Autodesk Inventor part; units mm, degrees
ref_plane "YZ Plane" through (0, 0, 0) normal (1, 0, 0) x (0, 1, 0)
ref_plane "XZ Plane" through (0, 0, 0) normal (0, 1, 0) x (-1, 0, 0)
ref_plane "XY Plane" through (0, 0, 0) normal (0, 0, 1) x (1, 0, 0)
sketch "Sketch1" plane through (0, 0, 0) normal (0, 0, 1) x (1, 0, 0)
  line L0 (30, -30) -> (30, 30)
  line L1 (30, 30) -> (-30, 30)
  line L2 (-30, 30) -> (-30, -30)
  line L3 (-30, -30) -> (30, 30) construction
  line L4 (30, -30) -> (-30, 30) construction
  line L5 (30, 30) -> (25, 30) construction
  line L6 (25, 30) -> (25, 25) construction
  line L7 (-30, 30) -> (-25, 30) construction
  line L8 (-25, 30) -> (-25, 25) construction
  line L9 (-30, -30) -> (-30, -25) construction
  line L10 (-30, -25) -> (-25, -25) construction
  line L11 (30, -30) -> (30, -25) construction
  line L12 (30, -25) -> (25, -25) construction
  circle A0 centre (-25, 25) radius 1.5
  circle A1 centre (25, 25) radius 1.5
  circle A2 centre (25, -25) radius 1.5
  circle A3 centre (-25, -25) radius 1.5
  line L13 (30, 30) -> (30, 18) construction
  line L14 (30, 18) -> (-30, 18)
  point P0 (0, 0)
  dimension "d0" = 60
  dimension "d1" = 60
  dimension "d2" = 5
  dimension "d3" = 5
  dimension "d4" = 5
  dimension "d5" = 5
  dimension "d6" = 5
  dimension "d7" = 5
  dimension "d8" = 5
  dimension "d9" = 5
  dimension "d10" = 3
  dimension "d11" = 3
  dimension "d12" = 3
  dimension "d13" = 3
  dimension "d46" = 12
sketch "Sketch1 outline for Block" plane through (0, 0, 0) normal (0, 0, 1) x (1, 0, 0)
  line L0 (30, 30) -> (30, 18)
  line L1 (-30, 30) -> (30, 30)
  line L2 (30, 18) -> (-30, 18)
  line L3 (-30, 18) -> (-30, 30)
  circle A0 centre (-25, 25) radius 1.5
  circle A1 centre (25, 25) radius 1.5
extrude "Block" add sketch "Sketch1 outline for Block" along normal blind 60
sketch "Sketch2" plane through (30, -30, 0) normal (1, 0, 0) x (0, 0, -1)
  line L0 (0, 60) -> (-60, 60)
  line L1 (-30, 60) -> (-12.75, 60)
  line L2 (-30, 60) -> (-47.25, 60)
  line L3 (-30, 60) -> (-30, 51.1) construction
  line L4 (-30, 51.1) -> (-6.75, 51.1)
  line L5 (-30, 51.1) -> (-53.25, 51.1)
  line L6 (-53.25, 51.1) -> (-53.25, 53.1)
  line L7 (-6.75, 51.1) -> (-6.75, 53.1)
  line L8 (-6.75, 53.1) -> (-12.75, 60)
  line L9 (-53.25, 53.1) -> (-47.25, 60)
  point P0 (0, 30)
  dimension "d17" = 17.25
  dimension "d18" = 17.25
  dimension "d19" = 8.9
  dimension "d20" = 23.25
  dimension "d21" = 23.25
  dimension "d22" = 2
  dimension "d23" = 2
sketch "Sketch2 outline for Tripod Slot" plane through (30, -30, 0) normal (1, 0, 0) x (0, 0, -1)
  line L0 (-12.75, 60) -> (-30, 60)
  line L1 (-6.75, 53.1) -> (-12.75, 60)
  line L2 (-6.75, 51.1) -> (-6.75, 53.1)
  line L3 (-30, 51.1) -> (-6.75, 51.1)
  line L4 (-53.25, 51.1) -> (-30, 51.1)
  line L5 (-53.25, 53.1) -> (-53.25, 51.1)
  line L6 (-47.25, 60) -> (-53.25, 53.1)
  line L7 (-30, 60) -> (-47.25, 60)
extrude "Tripod Slot" cut sketch "Sketch2 outline for Tripod Slot" against normal blind 60
sketch "Sketch3" plane through (0, 0, 60) normal (0, 0, 1) x (1, 0, 0)
  circle A0 centre (-25, -25) radius 1.5 construction
  line L0 (-25, -25) -> (-25, -20) construction
  line L1 (-25, -25) -> (-20, -25) construction
  line L2 (25.138807, -25) -> (25.138807, -20) construction
  line L3 (25.138807, -25) -> (30.138807, -25) construction
  line L4 (-25, 24.966147) -> (-25, 17.466147) construction
  line L5 (-25, 24.966147) -> (-17.5, 24.966147) construction
  line L6 (25.138807, 24.966147) -> (25.138807, 17.466147) construction
  line L7 (25.138807, 24.966147) -> (32.638807, 24.966147) construction
  line L8 (25.138807, 17.466147) -> (30, 17.466147) construction
  line L9 (30, 30) -> (30, 18) construction
  line L10 (-25, 17.466147) -> (-30, 17.466147) construction
  line L11 (-30, 30) -> (-30, 18) construction
  line L12 (-25, -20) -> (-30, -20) construction
  line L13 (25.138807, -20) -> (30, -20) construction
  line L14 (30, 17.466147) -> (5, 17.466147)
  line L15 (30, -20) -> (5, -20)
  line L16 (5, -20) -> (5, 17.466147)
  line L17 (-30, 17.466147) -> (-5, 17.466147)
  line L18 (-30, -20) -> (-5, -20)
  line L19 (-5, -20) -> (-5, 17.466147)
  line L20 (-30, 17.466147) -> (-30, -20)
  line L21 (30, 17.466147) -> (30, -20)
  point P0 (0, 0)
  point P1 (30, -30)
  point P2 (-30, -30)
  dimension "d26" = 5
  dimension "d27" = 90
  dimension "d28" = 5
  dimension "d29" = 90
  dimension "d30" = 7.5
  dimension "d31" = 90
  dimension "d32" = 7.5
  dimension "d33" = 90
  dimension "d34" = 25
  dimension "d35" = 25
  dimension "d36" = 25
  dimension "d37" = 25
  dimension "d38" = 90
  dimension "d39" = 90
  dimension "d40" = 4.86119
  dimension "d41" = 4.86119
  dimension "d42" = 55
sketch "Sketch3 outline for Plastic Thinning" plane through (0, 0, 60) normal (0, 0, 1) x (1, 0, 0)
  line L0 (30, -20) -> (30, 17.466147)
  line L1 (5, -20) -> (30, -20)
  line L2 (5, 17.466147) -> (5, -20)
  line L3 (30, 17.466147) -> (5, 17.466147)
  line L4 (-30, 17.466147) -> (-5, 17.466147)
  line L5 (-5, 17.466147) -> (-5, -20)
  line L6 (-5, -20) -> (-30, -20)
  line L7 (-30, -20) -> (-30, 17.466147)
extrude "Plastic Thinning" cut sketch "Sketch3 outline for Plastic Thinning" against normal blind 60
fillet "Strength" [suppressed]
fillet "Fillet3" radius 2 6 edges at (30, 18, 30) (30, 30, 6.375) (30, 30, 53.625) (-30, 18, 30) (-30, 30, 6.375) (-30, 30, 53.625)
sketch "Sketch4" plane through (-28, 18, 0) normal (0, -1, 0) x (1, 0, 0)
  line L0 (56, 60) -> (0, 60) construction
  line L1 (0, 0) -> (56, 0) construction
  line L2 (0, 60) -> (56, 0) construction
  circle A0 centre (28, 30) radius 11.25
  point P0 (28, 0)
  dimension "d48" = 22.5
sketch "Sketch4 outline for Extrusion4" plane through (-28, 18, 0) normal (0, -1, 0) x (1, 0, 0)
  circle A0 centre (28, 30) radius 11.25
extrude "Extrusion4" cut sketch "Sketch4 outline for Extrusion4" against normal blind 12.25
fillet "Fillet4" radius 2 2 edges at (-11.25, 21.1, 30) (-11.25, 18, 30)
properties part number "60x60CameraMountSlim"
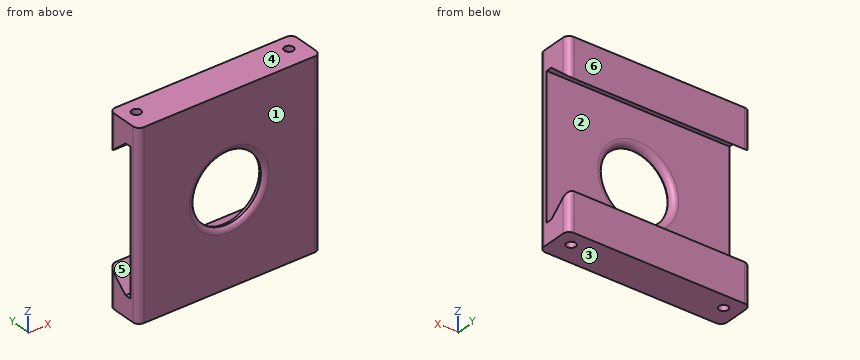
The listing builds one solid part. Answer for the finished solid, in the listing's coordinates (mm). Face numbers are marked on the shaded views. A direction names the side the tool comes from. Coordinates: 2 decimals unless noted, no trailing zeros. Write each loop counter-clockwise with the first axis right and the second up, starting at its lowest first coordinate (ties: lowest second). Pieces come first, ordered by that corner, then holes. Notation, with made-up numbers: (-22.75, 88.5) - (-1.75, 88.5) arc R17 ccw to (-1.75, 101.5) - close; hole circle Ø10 at (30, -0.75). An arc over 180 degrees is marked (long way). Return JSON: item names as keys, results as strings.
1. Which of the six approach directions +Z, -Z, +X, -X, +Y, -Y give full straight-line access (tool end or side, diameter ignored) to the marked faces 5 and 6?
Final values:
{"face 5": "+X, -X", "face 6": "+Z, -Z, +X, -X, +Y"}
2. The part is cut by section C-C on y = 25. Determine the outline of the cut face in (x, z).
Final values:
{"outline": "(-30, 0) - (-26.5, 0) - (-26.5, 8.4) - (-30, 8.4) - close; (-30, 51.6) - (-26.5, 51.6) - (-26.5, 60) - (-30, 60) - close; (-23.5, 0) - (23.5, 0) - (23.5, 8.4) - (-23.5, 8.4) - close; (-23.5, 51.6) - (23.5, 51.6) - (23.5, 60) - (-23.5, 60) - close; (26.5, 0) - (30, 0) - (30, 8.4) - (26.5, 8.4) - close; (26.5, 51.6) - (30, 51.6) - (30, 60) - (26.5, 60) - close"}
3. For a pull along Z with two mould halves and no side action, classify the marked faces 1, 2, 3 and 4 as +Z half, -Z half, draft (parallel to the pull), parting line (faces both ways), or undercut.
Final values:
{"face 1": "draft", "face 2": "undercut", "face 3": "-Z half", "face 4": "+Z half"}
4. The part is cut by section A-A on z = 5. Determine the outline of the cut face in (x, y), then the cut area to 3 significant figures.
Final values:
{"outline": "(-30, 20) arc R2 ccw to (-28, 18) - (28, 18) arc R2 ccw to (30, 20) - (30, 28) arc R2 ccw to (28, 30) - (-28, 30) arc R2 ccw to (-30, 28) - close; hole circle Ø3 at (-25, 25); hole circle Ø3 at (25, 25)", "area": "702 mm^2"}
5. Each of these flat-tipped pins is pushed along its axis until it touches: pin 1 Ø10 at (x, z) = (-13, 40.5) entering from +Y; pin 2 Ø2.5 at (x, y) = (-25, 25) entering from +Z. Where does it stop, or does it pass through?
Final values:
{"pin 1": "y = 21.1", "pin 2": "through"}
6. The part is cut by section B-B on x = 25. Determine the outline of the cut face in (y, z).
Final values:
{"outline": "(18, 0) - (23.5, 0) - (23.5, 7.1) - (23.1, 6.75) - (21.1, 6.75) - (21.1, 53.25) - (23.1, 53.25) - (23.5, 52.9) - (23.5, 60) - (18, 60) - close; (26.5, 0) - (30, 0) - (30, 12.75) - (26.5, 9.71) - close; (26.5, 50.29) - (30, 47.25) - (30, 60) - (26.5, 60) - close"}
7. Consider line 1 along X through (y, z) = (25, 5.5); line 2 along Z through (x, y) = (-3, 26.5); line 3 along X through (y, z) = (26.25, 53). Determine where each line is inside the solid, lowest interval first.
Final values:
{"line 1": "-30 to -26.5, -23.5 to 23.5, 26.5 to 30", "line 2": "0 to 9.71, 50.29 to 60", "line 3": "-30 to -25.83, -24.17 to 24.17, 25.83 to 30"}
